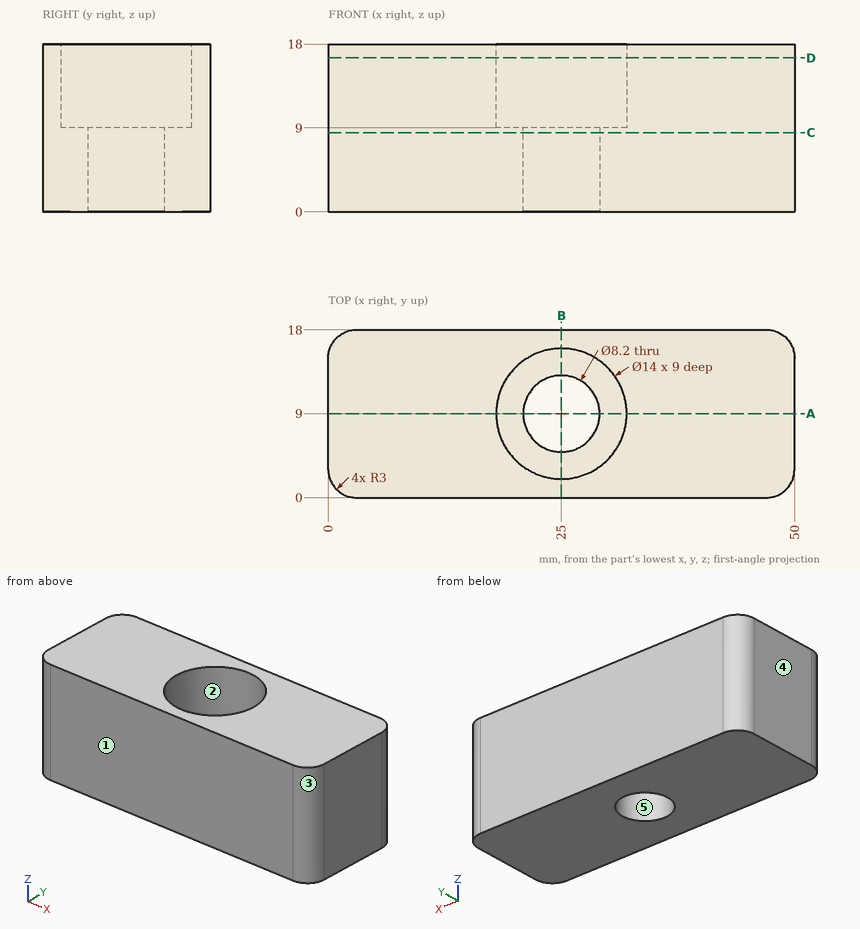
Answer from the drawing. Dimensions are ordinates in mm from the lowest x, y and z of the part. A direction names the side the tool comes from. Coordinates: 2 decimals unless noted, no trailing zeros. Write each loop counter-clockwise with the first axis right and the second up, starting at its lowest first coordinate (ties: lowest second). Pieces come first, ordered by that corner, then holes. Notation, with made-up numbers: M -10.75,-31 L 40.25,-31 A16 cw 40.25,-20 Z; hole C -14.5,64 d7. An arc over 180 degrees is marked long. Use a Markdown table: item, result.
Q1. Determine the mould class of the marked faces 3, 4 and 5 for opening direction Y: released by +Y, released by -Y, zero draft, split by the parting line, or undercut.
Answer block:
| item | result |
|---|---|
| face 3 | released by -Y |
| face 4 | zero draft |
| face 5 | undercut |
Q2. Which of the six approach directions +Z, -Z, +X, -X, +Y, -Y give full straight-line access (tool end or side, diameter ignored) to the marked faces 1 and 2?
Answer block:
| item | result |
|---|---|
| face 1 | +Z, -Z, +X, -X, -Y |
| face 2 | +Z |
Q3. The part is cut by section A-A, the plane y = 9. Write down the section's boundary in (x, z), then the cut area to 3 significant figures.
Answer block:
| item | result |
|---|---|
| outline | M 0,0 L 20.9,0 L 20.9,9 L 18,9 L 18,18 L 0,18 Z; M 29.1,0 L 50,0 L 50,18 L 32,18 L 32,9 L 29.1,9 Z |
| area | 700 mm2 |
Q4. Straight lines are drawn through the part: L1, parallel to Y at x = 25, z = 5.25; L2, parallel to Y at x = 25, z = 15.25; L3, parallel to X at y = 4, z = 9.25. For each, find the intervals that lie inside material, in ascending order. Write a range as [from, to].
Answer block:
| item | result |
|---|---|
| L1 | y = [0, 4.9], [13.1, 18] |
| L2 | y = [0, 2], [16, 18] |
| L3 | x = [0, 20.1], [29.9, 50] |
Q5. The part is cut by section B-B, the plane x = 25. Write down the section's boundary in (y, z).
Answer block:
| item | result |
|---|---|
| outline | M 0,0 L 4.9,0 L 4.9,9 L 2,9 L 2,18 L 0,18 Z; M 13.1,0 L 18,0 L 18,18 L 16,18 L 16,9 L 13.1,9 Z |
Q6. The part is cut by section D-D, the plane z = 16.5. Write down the section's boundary in (x, y), then the cut area to 3 significant figures.
Answer block:
| item | result |
|---|---|
| outline | M 0,3 A3 ccw 3,0 L 47,0 A3 ccw 50,3 L 50,15 A3 ccw 47,18 L 3,18 A3 ccw 0,15 Z; hole C 25,9 d14 |
| area | 738 mm2 |
Q7. The part is cut by section C-C, the plane z = 8.5. Write down the section's boundary in (x, y).
Answer block:
| item | result |
|---|---|
| outline | M 0,3 A3 ccw 3,0 L 47,0 A3 ccw 50,3 L 50,15 A3 ccw 47,18 L 3,18 A3 ccw 0,15 Z; hole C 25,9 d8.2 |
Q8. This flat-tipped pin is pushed along its axis until it touches: pin 1 Ø4 at (x, y) = (24.5, 6) entering from +Z. Where does it stop, or does it pass through?
Answer block:
| item | result |
|---|---|
| pin 1 | stops at z = 9 |
